For this review, take the finished solid that the model builds, in its own axes (mm). Face numbers are marked on the shaded views. A direction names the side the tool comes from. Coordinates: 2 decimals unless noted, no trailing zeros. Loops run counter-clockwise (first coordinate to the right, second up) from the corner with the lowest first, then second, coordinate; pieces in that order, holes last. Notation, with made-up numbers: M -16,59 L 3,59 A30 ccw 3,85 Z; hole C 39,-8 d8. An arc over 180 degrees is marked long. Put each result on its own line as item: value.
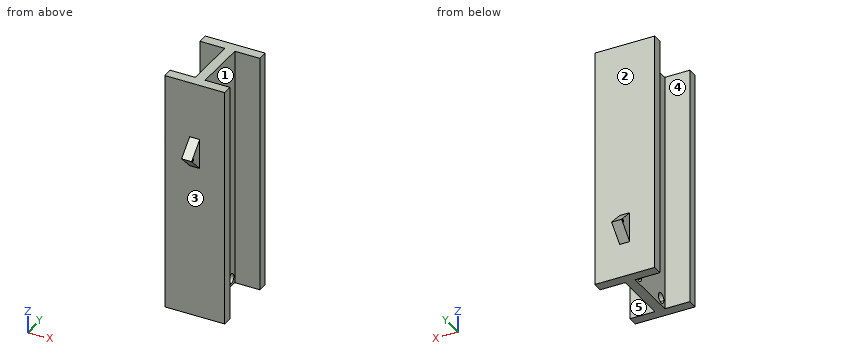
```python
from build123d import *

# Parameters (mm, degrees)
BOSS_EXTRUDE1_DEPTH      = 1219.2
BOSS_EXTRUDE2_DEPTH      = 0.072177487
BOSS_EXTRUDE2_DEPTH_BACK = 50.872177487
BOSS_EXTRUDE3_DEPTH      = 0.072177487
BOSS_EXTRUDE3_DEPTH_BACK = 50.872177487
CUT_EXTRUDE1_DEPTH       = 101.6
CUT_EXTRUDE1_DEPTH_BACK  = 101.6
CUT_EXTRUDE3_DEPTH       = 76.2
CUT_EXTRUDE3_DEPTH_BACK  = 76.2
SKETCH7_R                = 6.35


with BuildPart() as part:
    # Sketch1 → Boss-Extrude1 (new body)
    with BuildSketch(Plane.XY):
        Polygon((152.4, 190.5), (-152.4, 190.5), (-152.4, 139.7), (-25.4, 139.7), (-25.4, -139.7), (-152.4, -139.7), (-152.4, -190.5), (152.4, -190.5), (152.4, -139.7), (25.4, -139.7), (25.4, 139.7), (152.4, 139.7), align=None)
    extrude(amount=BOSS_EXTRUDE1_DEPTH)

    # Sketch3 → Boss-Extrude2 (add, two sides: drawn at the far end of the back side and taken through both)
    with BuildSketch(Plane(origin=(25.4, 0, 0), x_dir=(0, 0, -1), z_dir=(1, 0, 0)).offset(-BOSS_EXTRUDE2_DEPTH_BACK)):
        Polygon((-325.848703736, 190.5), (-249.681440183, 190.5), (-249.681440183, 266.7), align=None)
        Polygon((-249.681440183, 266.7), (-249.681440183, 190.5), (-173.448689666, 190.5), align=None)
    extrude(amount=BOSS_EXTRUDE2_DEPTH + BOSS_EXTRUDE2_DEPTH_BACK)

    # Sketch4 → Boss-Extrude3 (add, two sides: drawn at the far end of the back side and taken through both)
    with BuildSketch(Plane(origin=(25.4, 0, 0), x_dir=(0, 0, -1), z_dir=(1, 0, 0)).offset(-BOSS_EXTRUDE3_DEPTH_BACK)):
        Polygon((-859.248696701, -266.7), (-859.248696701, -190.5), (-934.329981547, -190.5), align=None)
        Polygon((-781.913312631, -190.5), (-859.248696701, -190.5), (-859.248696701, -266.7), align=None)
    extrude(amount=BOSS_EXTRUDE3_DEPTH + BOSS_EXTRUDE3_DEPTH_BACK)

    # Sketch6 → Cut-Extrude1 (cut, two sides: drawn at the far end of the back side and taken through both)
    with BuildSketch(Plane(origin=(25.4, 0, 0), x_dir=(0, 0, -1), z_dir=(1, 0, 0)).offset(-CUT_EXTRUDE1_DEPTH_BACK)):
        with BuildLine():
            ThreePointArc((-38.1, 79.375), (-20.139487758, 86.814487758), (-12.7, 104.775))
            Line((-12.7, 104.775), (-38.1, 104.775))
            Line((-38.1, 104.775), (-38.1, 79.375))
        make_face()
        with BuildLine():
            Line((-38.1, 104.775), (-12.7, 104.775))
            ThreePointArc((-12.7, 104.775), (-56.060512242, 122.735512242), (-38.1, 79.375))
            Line((-38.1, 79.375), (-38.1, 104.775))
        make_face()
        with BuildLine():
            Line((-38.1, -130.175), (-38.1, -104.775))
            Line((-38.1, -104.775), (-38.1, -79.375))
            ThreePointArc((-38.1, -79.375), (-63.5, -104.775), (-38.1, -130.175))
        make_face()
        with BuildLine():
            ThreePointArc((-38.1, -130.175), (-20.139487758, -122.735512242), (-12.7, -104.775))
            Line((-12.7, -104.775), (-38.1, -104.775))
            Line((-38.1, -104.775), (-38.1, -130.175))
        make_face()
        with BuildLine():
            Line((-38.1, -104.775), (-12.7, -104.775))
            ThreePointArc((-12.7, -104.775), (-20.139487758, -86.814487758), (-38.1, -79.375))
            Line((-38.1, -79.375), (-38.1, -104.775))
        make_face()
    extrude(amount=CUT_EXTRUDE1_DEPTH + CUT_EXTRUDE1_DEPTH_BACK, mode=Mode.SUBTRACT)

    # Sketch7 → Cut-Extrude3 (cut, two sides: drawn at the far end of the back side and taken through both)
    with BuildSketch(Plane(origin=(25.472177487, 0, 0), x_dir=(0, 0, -1), z_dir=(1, 0, 0)).offset(-CUT_EXTRUDE3_DEPTH_BACK)):
        with Locations(Location((-249.681440183, 254, 0), (0, 0, 180))):
            Circle(SKETCH7_R)
        with Locations(Location((-859.248696701, -254, 0), (0, 0, 180))):
            Circle(SKETCH7_R)
    extrude(amount=CUT_EXTRUDE3_DEPTH + CUT_EXTRUDE3_DEPTH_BACK, mode=Mode.SUBTRACT)


solid = part.part
```
(1) For pin 1 (1 mm diameter, centred on x = -35.5, z = 206.5, fed in from -Y); pin 2 (1.5 mm diameter, centred on y = -49.5, z = 976.5, fed in from -X); pin 3 (2 mm diameter, centred on x = 18, y = -18, fed in from -Z); pin 4 (8 mm diameter, centred on y = 43.5, z = 1010.5, fed in from +X), all flat-tipped, find the tip position at first contact; note any pin that passes through.
Determined:
pin 1: stops at y = -190.5
pin 2: stops at x = -25.4
pin 3: stops at z = 0
pin 4: stops at x = 25.4
(2) Tool access review of the marked faces 4 and 5: name each direction out of +Z, -Z, +X, -X, +Y, -Y from which nothing blocks a thin tool from reaching the whole face with its end or side.
Determined:
face 4: +Z, -Z, -X
face 5: +Z, -Z, +X
(3) Wall thickness on line 1 along Y through (x, z) = (9, 38); line 2 along Y through (x, z) = (91.5, 1124); line 3 along X through (y, z) = (-18, 935): over which ranges is each line inside the solid? List them lowest first. Write a range as [from, to].
Determined:
line 1: y = [-190.5, -130.17], [-79.38, 79.38], [130.17, 190.5]
line 2: y = [-190.5, -139.7], [139.7, 190.5]
line 3: x = [-25.4, 25.4]
(4) Add section C-C (y = -8.5). Write out the cut boundary in (x, z), plus the area to 3 significant figures.
Determined:
outline: M -25.4,0 L 25.4,0 L 25.4,1219.2 L -25.4,1219.2 Z
area: 61,900 mm^2
(5) Add section A-A (x = 48.5). Write out the cut boundary in (y, z), plus the area to 3 significant figures.
Determined:
outline: M -190.5,0 L -139.7,0 L -139.7,1219.2 L -190.5,1219.2 Z; M 139.7,0 L 190.5,0 L 190.5,1219.2 L 139.7,1219.2 Z
area: 124,000 mm^2
(6) Add section B-B (z = 725.5). Write out the cut boundary in (x, y), plus the area to 3 significant figures.
Determined:
outline: M -152.4,-190.5 L 152.4,-190.5 L 152.4,-139.7 L 25.4,-139.7 L 25.4,139.7 L 152.4,139.7 L 152.4,190.5 L -152.4,190.5 L -152.4,139.7 L -25.4,139.7 L -25.4,-139.7 L -152.4,-139.7 Z
area: 45,200 mm^2
(7) Draft analysis for pull direction Y (two halves, no side actions). For the marked faces 1, 2 and 3, state which applies: +Y half, -Y half, draft (parallel to the pull), parting line (faces both ways), or undercut.
Determined:
face 1: undercut
face 2: +Y half
face 3: -Y half
